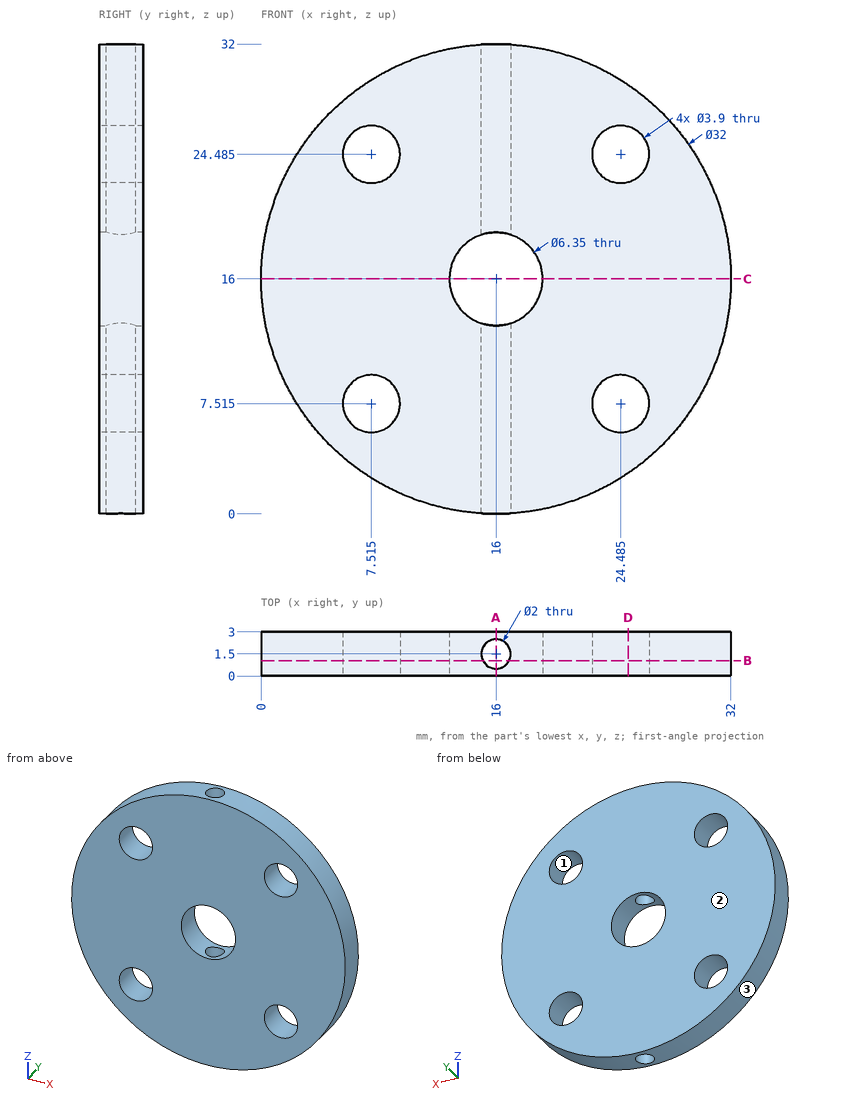
For this review, use the dimensioned drawing (mm, ordinates from the lowest corner) and the shaded views. Coordinates: 2 decimals unless noted, no trailing zeros. Loops run counter-clockwise (first coordinate to the right, second up) from the corner with the lowest first, then second, coordinate; pieces in that order, holes last. Notation, with made-up numbers: (41, 44) -> (81, 44) arc R28 ccw to (81, 77) -> close; hole circle Ø3 at (23.25, 14.25). An arc over 180 degrees is marked (long way). Write each question's results on one line, items separated by ' | '.
Q1. Add section C-C, the plane z = 16. State the section outline as (x, y) points (1 decimal).
Taken from the geometry:
outline: (0, 0) -> (12.8, 0) -> (12.8, 3) -> (0, 3) -> close; (19.2, 0) -> (32, 0) -> (32, 3) -> (19.2, 3) -> close
Q2. To check wall thickness, follow line 1 along Z through (x, y) = (9, 0.4); line 2 along X through (y, z) = (0.85, 7) (1 decimal); line 3 along Z through (x, y) = (7, 0.9) (1 decimal). State the ranges of each line that lie inside material, in increasing order. Write a range as [from, to].
Taken from the geometry:
line 1: [1.61, 6.25], [8.78, 23.22], [25.75, 30.39] | line 2: [2.8, 5.6], [9.4, 15.2], [16.8, 22.6], [26.4, 29.2] | line 3: [2.8, 5.6], [9.4, 22.6], [26.4, 29.2]
Q3. Add section B-B, the plane y = 1.05. Count the separate pieces of the cut face and the enclosed holes in it, then the cut area to 3 significant figures.
Taken from the geometry:
separate pieces: 2 | enclosed holes: 4 | area: 679 mm²
Q4. Add section D-D, the plane x = 25. State the section outline as (y, z) points (1 decimal), then the cut area to 3 significant figures.
Taken from the geometry:
outline: (0, 2.8) -> (3, 2.8) -> (3, 5.6) -> (0, 5.6) -> close; (0, 9.4) -> (3, 9.4) -> (3, 22.6) -> (0, 22.6) -> close; (0, 26.4) -> (3, 26.4) -> (3, 29.2) -> (0, 29.2) -> close | area: 56.8 mm²
Q5. Add section A-A, the plane x = 16. State the section outline as (y, z) points (1 decimal).
Taken from the geometry:
outline: (0, 0) -> (0.5, 0) -> (0.5, 12.8) -> (0, 12.8) -> close; (0, 19.2) -> (0.5, 19.2) -> (0.5, 32) -> (0, 32) -> close; (2.5, 0) -> (3, 0) -> (3, 12.8) -> (2.5, 12.8) -> close; (2.5, 19.2) -> (3, 19.2) -> (3, 32) -> (2.5, 32) -> close
Q6. Mouldability with a two-part tool opening along Z and no side actions: class the marked faces 1, 2 and 3 as +Z half, -Z half, draft (parallel to the pull), parting line (faces both ways), or undercut.
Taken from the geometry:
face 1: undercut | face 2: draft | face 3: parting line
